Build history of the part. All positions in model axes, mm. A direction names the side the tool comes from. Give positions to 0.01 mm unless a question says otherwise; leave off trailing zeros. Order: outer loops, then holes, each group sorted by start corner. A loop starts at its lowest first (then second) coordinate and runs counter-clockwise, first axis right, second up. Notation, with made-up numbers: (-22, 87) - (36, 87) arc R21 cw to (36, 94) - close; hole circle Ø9 at (83, 68). An arc over 180 degrees is marked (long way). Answer in a Markdown table with one row per item.
```python
from build123d import *

# Parameters (mm, degrees)
SKETCH1_W               = 80
SKETCH1_H               = 36
BOSS_EXTRUDE1_DEPTH     = 1.6
SKETCH2_W               = 69.34
SKETCH2_H               = 24.3
BOSS_EXTRUDE2_DEPTH     = 7.32
BOSS_EXTRUDE3_DEPTH     = 3.46
CUT_EXTRUDE1_DEPTH      = 45.470016865
CUT_EXTRUDE1_DEPTH_BACK = 45.470016865
SKETCH4_R               = 1.36


with BuildPart() as part:
    # Sketch1 → Boss-Extrude1 (new body)
    with BuildSketch(Plane(origin=(0, 0, 0), x_dir=(1, 0, 0), z_dir=(0, 1, 0))):
        Rectangle(SKETCH1_W, SKETCH1_H)
    extrude(amount=BOSS_EXTRUDE1_DEPTH)

    # Sketch2 → Boss-Extrude2 (add)
    with BuildSketch(Plane(origin=(0, 1.6, 0), x_dir=(1, 0, 0), z_dir=(0, 1, 0))):
        with Locations((0.13, -0.59)):
            Rectangle(SKETCH2_W, SKETCH2_H)
    extrude(amount=BOSS_EXTRUDE2_DEPTH)

    # Sketch3 → Boss-Extrude3 (add)
    with BuildSketch(Plane(origin=(0, 1.6, 0), x_dir=(1, 0, 0), z_dir=(0, 1, 0))):
        Polygon((40, 5.66), (40, -6.84), (37.4, -9.74), (34.8, -9.74), (34.8, 8.56), (37.4, 8.56), align=None)
    extrude(amount=BOSS_EXTRUDE3_DEPTH)

    # Sketch4 → Cut-Extrude1 (cut, two sides: drawn at the far end of the back side and taken through both)
    with BuildSketch(Plane(origin=(0, 1.6, 0), x_dir=(1, 0, 0), z_dir=(0, 1, 0)).offset(-CUT_EXTRUDE1_DEPTH_BACK)):
        with Locations(Location((-37.5, 15.5, 0), (0, 0, 270))):
            Circle(SKETCH4_R)
        with Locations(Location((-37.5, -15.5, 0), (0, 0, 270))):
            Circle(SKETCH4_R)
        with Locations(Location((37.5, -15.5, 0), (0, 0, 270))):
            Circle(SKETCH4_R)
        with Locations(Location((37.5, 15.5, 0), (0, 0, 270))):
            Circle(SKETCH4_R)
    extrude(amount=CUT_EXTRUDE1_DEPTH + CUT_EXTRUDE1_DEPTH_BACK, mode=Mode.SUBTRACT)


solid = part.part
```
1. Cut at B-B on x = -37.5. Write the cut outline in (y, z).
Check result:
| item | result |
|---|---|
| outline | (0, -18) - (1.6, -18) - (1.6, -16.86) - (0, -16.86) - close; (0, -14.14) - (1.6, -14.14) - (1.6, 14.14) - (0, 14.14) - close; (0, 16.86) - (1.6, 16.86) - (1.6, 18) - (0, 18) - close |
2. Drop flat-ended pins along their axis: P1, Ø2.5, axis at x = -37.5, z = 15.5, coming from the +Y side; P2, Ø2, axis at x = 19, y = 3, coming from the +Z side; P3, Ø3.5, axis at x = 4, y = 6.5, coming from the -Z side; P4, Ø2, axis at x = 36.5, y = 3.5, coming from the -Z side. Give the stop position or say it passes through.
Check result:
| item | result |
|---|---|
| P1 | passes through |
| P2 | stops at z = 12.74 |
| P3 | stops at z = -11.56 |
| P4 | stops at z = -8.56 |
3. Cut at D-D on z = 0.5. Write the cut outline in (x, y), and give its area (3 significant figures).
Check result:
| item | result |
|---|---|
| outline | (-40, 0) - (40, 0) - (40, 5.06) - (34.8, 5.06) - (34.8, 8.92) - (-34.54, 8.92) - (-34.54, 1.6) - (-40, 1.6) - close |
| area | 654 mm² |
4. Probe line 1 (Z direction, x = -37.5, y = 1.15); line 2 (X direction, y = 1.25, z = 15.5); line 3 (Y direction, x = 33, z = -14). List the from-to ranges inside material, lowest first.
Check result:
| item | result |
|---|---|
| line 1 | z = -18 to -16.86, -14.14 to 14.14, 16.86 to 18 |
| line 2 | x = -40 to -38.86, -36.14 to 36.14, 38.86 to 40 |
| line 3 | y = 0 to 1.6 |
5. Cut at A-A on z = -15.5. Write the cut outline in (x, y).
Check result:
| item | result |
|---|---|
| outline | (-40, 0) - (-38.86, 0) - (-38.86, 1.6) - (-40, 1.6) - close; (-36.14, 0) - (36.14, 0) - (36.14, 1.6) - (-36.14, 1.6) - close; (38.86, 0) - (40, 0) - (40, 1.6) - (38.86, 1.6) - close |
6. Two-plate mould, pull along X, no slides. Class faces 1 (the face through (37, 5.06, 0)), 2 (the face through (38.647, 0.789, -14.769)), 3 (the face through (40, 2, 0)), 4 (the face through (-34.54, 5, 1)): +X half, -X half, draft (parallel to the pull), parting line (faces both ways), or undercut.
Check result:
| item | result |
|---|---|
| face 1 | draft |
| face 2 | undercut |
| face 3 | +X half |
| face 4 | -X half |
7. Which spindle directions (+Z, -Z, +X, -X, +Y, -Y) get a long thin tool onto all of the face, cutting with end or side? Do faces 5 (the face through (0, 5, -11.56)), 6 (the face through (36, 3, 9.74)), 7 (the face through (36, 3, -8.56)). Say none if no direction does.
Check result:
| item | result |
|---|---|
| face 5 | -Z, +X, -X, +Y |
| face 6 | +Z, +X, +Y |
| face 7 | -Z, +X, +Y |
8. Cut at C-C on x = 13. Write the cut outline in (y, z).
Check result:
| item | result |
|---|---|
| outline | (0, -18) - (1.6, -18) - (1.6, -11.56) - (8.92, -11.56) - (8.92, 12.74) - (1.6, 12.74) - (1.6, 18) - (0, 18) - close |
